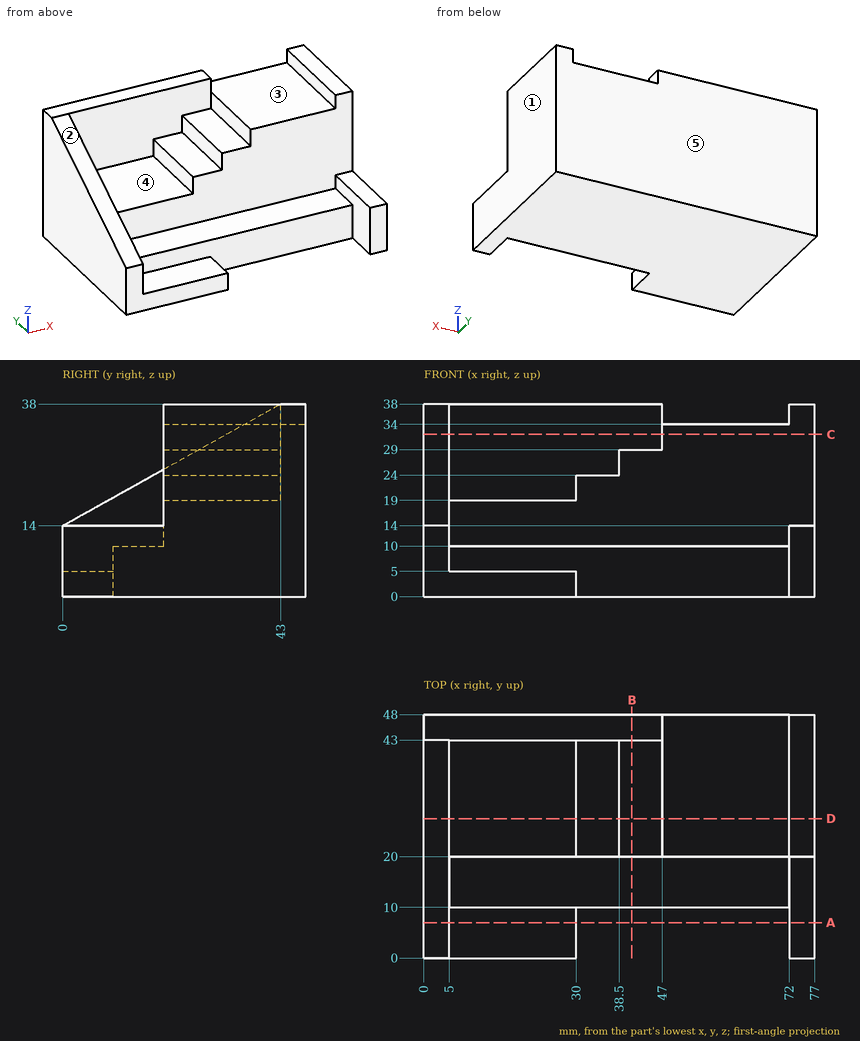
Source: three-view drawing plus pictorial views. Frame: mm from the lowest corner of the part. A direction names the side the tool comes from. Give positions to 0.01 mm unless a question says otherwise; leave off trailing zeros. Order: outer loops, then holes, each group sorted by start corner. A loop starts at its lowest first (then second) coordinate and runs counter-clockwise, first axis right, second up.
1. Reachability of the marked faces 1, 2, 3, 4 and 5 from +Z, -Z, +X, -X, +Y, -Y: full face, straight path, thin tool, end or side. Return the list, or none.
Derived:
face 1: +Z, -Z, +X, +Y, -Y
face 2: +Z, -X, -Y
face 3: +Z, +Y, -Y
face 4: +Z, -Y
face 5: +Z, -Z, +X, -X, +Y
2. Section D-D on y = 27.5. Return the cut outline in (x, z).
Derived:
outline: (0, 0) - (77, 0) - (77, 38) - (72, 38) - (72, 34) - (47, 34) - (47, 29) - (38.5, 29) - (38.5, 24) - (30, 24) - (30, 19) - (5, 19) - (5, 29.35) - (0, 29.35) - close
3. Material intervals for L1, parallel to X at y = 8, z = 13; L2, parallel to Z at x = 56.5, y = 17; L3, parallel to Y at x = 32.5, z = 12, sorted ascending.
Derived:
L1: x = 0 to 5, 72 to 77
L2: z = 0 to 10
L3: y = 20 to 48
4. Section C-C on z = 32. Return the cut outline in (x, y).
Derived:
outline: (0, 32.25) - (5, 32.25) - (5, 43) - (47, 43) - (47, 20) - (77, 20) - (77, 48) - (0, 48) - close
5. Section A-A on y = 7. Return the cut outline in (x, z), and give its area (3 significant figures).
Derived:
outline: (0, 0) - (30, 0) - (30, 5) - (5, 5) - (5, 17.91) - (0, 17.91) - close; (72, 0) - (77, 0) - (77, 14) - (72, 14) - close
area: 285 mm2
6. Section B-B on x = 41. Return the cut outline in (y, z).
Derived:
outline: (10, 0) - (48, 0) - (48, 38) - (43, 38) - (43, 29) - (20, 29) - (20, 10) - (10, 10) - close
7. Pin query (flat end, axial travel): pin 1 (12.5 mm diameter, centred on x = 65, y = 29, fed in from +Z); pin 2 (2.5 mm diameter, centred on x = 44.5, y = 30.5, fed in from +Z); pin 3 (11 mm diameter, centred on x = 22.5, y = 3.5, fed in from +Z). Return the tip coordinate at first contact, or that it passes through.
Derived:
pin 1: stops at z = 34
pin 2: stops at z = 29
pin 3: stops at z = 5
